from build123d import *

# Parameters (mm, degrees)
F0_R          = 51
F0_R_2        = 2.5
F1_DEPTH      = 8
F1_DEPTH_BACK = 7
F2_R          = 57.85
F2_R_2        = 55.35
F3_DEPTH      = 3


with BuildPart() as f1:
    # F0 (on Front) → F1 (new body, two sides)
    with BuildSketch(Plane.XZ) as f1_sk:
        Circle(F0_R)
        with Locations((-21.5, -37.239092)):
            Circle(F0_R_2, mode=Mode.SUBTRACT)
        with Locations((-21.5, 37.239092)):
            Circle(F0_R_2, mode=Mode.SUBTRACT)
        with BuildLine():
            ThreePointArc((2.041061, 4.902058), (3.356125, 4.114915), (4.391594, 2.984962))
            ThreePointArc((4.391594, 2.984962), (5.075208, 1.561527), (5.31, 0))
            ThreePointArc((5.31, 0), (5.075312, -1.561189), (4.391992, -2.984377))
            ThreePointArc((4.391992, -2.984377), (3.469883, -4.019454), (2.311288, -4.780591))
            ThreePointArc((2.311288, -4.780591), (-0.462852, -5.289789), (-3.106405, -4.306547))
            ThreePointArc((-3.106405, -4.306547), (-3.356125, -4.114915), (-3.594051, -3.908823))
            ThreePointArc((-3.594051, -3.908823), (-5.088714, -1.516936), (-5.147666, 1.302933))
            ThreePointArc((-5.147666, 1.302933), (-4.635012, 2.5909), (-3.806465, 3.702286))
            ThreePointArc((-3.806465, 3.702286), (-1.067252, 5.201641), (2.041061, 4.902058))
        make_face(mode=Mode.SUBTRACT)
        with Locations((43, 0)):
            Circle(F0_R_2, mode=Mode.SUBTRACT)
    extrude(amount=F1_DEPTH)
    extrude(f1_sk.sketch, amount=-F1_DEPTH_BACK)

    # F2 (on face) → F3 (cut)
    with BuildSketch(Plane(origin=(0, 7, 0), x_dir=(-1, 0, 0), z_dir=(0, 1, 0))):
        Circle(F2_R)
        Circle(F2_R_2, mode=Mode.SUBTRACT)
    extrude(amount=-F3_DEPTH, mode=Mode.SUBTRACT)


solid = f1.part
Read the model definition and answer for the solid it produces. Units are mm, in the model's axes. Round coordinates to 2 decimals unless told otherwise and drop trailing zeros. Loops run counter-clockwise (first coordinate to the right, second up) from the corner with the lowest first, then second, coordinate; pieces in that order, holes last. Notation, with made-up numbers: (85.25, 48) - (133.25, 48) arc R19 cw to (133.25, 68) - close; hole circle Ø2 at (80.5, 60.25). An arc over 180 degrees is marked (long way). One line per question, with ' | ' between items. Start each with the question number.
Q1. For a pull along X with two mould halves and no side action, classify faces 1 (the cylindrical face through (-11.056, -0.605, -49.787)), 2 (the flat face through (-1, -8, -11)), 3 (the cylindrical face through (-23.34, -0.39, 38.93)) as +X half, -X half, draft (parallel to the pull), parting line (faces both ways), or undercut.
Q2. Flat-ended cylindrical pins translate along their axes: pin 1 (3 mm diameter, centred on x = 17.5, y = 0, fed in from +Z); pin 2 (3 mm diameter, centred on y = 1.5, z = 14, fed in from +X); pin 3 (4 mm diameter, centred on x = -36, y = 0.5, fed in from +Z). Find the tip coordinate at first contact, or state that the pin passes through.
Q3. Section C-C on x = -21.5 is taken. Give the vertices of the cut face in (y, z), plus the area to 3 significant figures.
Q4. Find the intervals of material crossed by L1, parallel to Z at x = -22.5, y = -6.5; L2, parallel to Z at x = -21.5, y = 1; L3, parallel to Z at x = -1.5, y = 2, in increasing order.
Q5. Section A-A on x = 0 is taken. Give the vertices of the cut face in (y, z).
Q6. Section B-B on y = 5.75 is taken. Give the vertices of the cut face in (x, z).
Q7. Section D-D on z = -42 is taken. Give the vertices of the cut face in (x, y).
Established:
1) face 1: parting line | face 2: draft | face 3: undercut
2) pin 1: z = 48.43 | pin 2: x = 49.44 | pin 3: z = 38.01
3) outline: (-8, -46.25) - (7, -46.25) - (7, -39.74) - (-8, -39.74) - close; (-8, -34.74) - (7, -34.74) - (7, 34.74) - (-8, 34.74) - close; (-8, 39.74) - (7, 39.74) - (7, 46.25) - (-8, 46.25) - close | area: 1,240 mm²
4) L1: -45.77 to -39.53, -34.95 to 34.95, 39.53 to 45.77 | L2: -46.25 to -39.74, -34.74 to 34.74, 39.74 to 46.25 | L3: -50.98 to -5.09, 5.09 to 50.98
5) outline: (-8, -51) - (7, -51) - (7, -5.31) - (-8, -5.31) - close; (-8, 5.31) - (7, 5.31) - (7, 51) - (-8, 51) - close
6) outline: circle Ø102 at (0, 0); hole circle Ø5 at (-21.5, -37.24); hole circle Ø5 at (-21.5, 37.24); hole (-5.15, 1.3) arc R5.31 ccw to (-3.59, -3.91) arc R5.31 ccw to (-3.11, -4.31) arc R5.31 ccw to (2.31, -4.78) arc R5.31 ccw to (4.39, -2.98) arc R5.31 ccw to (5.31, 0) arc R5.31 ccw to (4.39, 2.98) arc R5.31 ccw to (2.04, 4.9) arc R5.31 ccw to (-3.81, 3.7) arc R5.31 ccw to start; hole circle Ø5 at (43, 0)
7) outline: (-28.93, -8) - (28.93, -8) - (28.93, 7) - (-28.93, 7) - close
